For this review, take the finished solid that the model builds, in its own axes (mm). Give positions to 0.01 mm unless a question says otherwise; leave off trailing zeros. Write each loop counter-clockwise with the first axis right and the second up, starting at its lowest first coordinate (ties: lowest second). Pieces come first, ordered by that corner, then holes. Notation, with made-up numbers: M -30.75,37.25 L -25.75,37.25 A25 ccw -25.75,49.25 Z; hole C 39.25,-35 d7. An arc over 180 degrees is marked long. Write item = value, one per line.
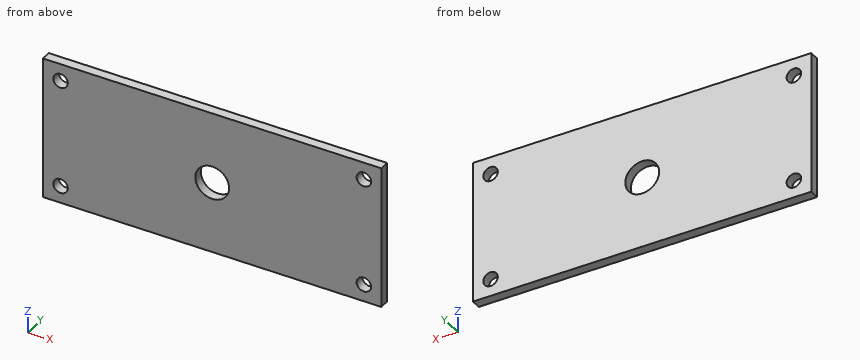
```python
from build123d import *

# Parameters (mm, degrees)
F0_W     = 70
F0_H     = 30
F1_DEPTH = 2
F2_R     = 1.5
F3_DEPTH = 25
F4_R     = 3.5
F5_DEPTH = 2.001


with BuildPart() as f1:
    # F0 (on Front) → F1 (new body)
    with BuildSketch(Plane.XZ):
        Rectangle(F0_W, F0_H)
    extrude(amount=F1_DEPTH)

    # F2 (on face) → F3 (cut)
    with BuildSketch(Plane.XZ.offset(2)):
        with Locations((-31.372793, 11.372793)):
            Circle(F2_R)
        with Locations((31.372793, 11.372793)):
            Circle(F2_R)
        with Locations((-31.372793, -11.372793)):
            Circle(F2_R)
        with Locations((31.372793, -11.372793)):
            Circle(F2_R)
    extrude(amount=-F3_DEPTH, mode=Mode.SUBTRACT)

    # F4 (on face) → F5 (cut, through all)
    with BuildSketch(Plane.XZ.offset(2)):
        Circle(F4_R)
    extrude(amount=-F5_DEPTH, mode=Mode.SUBTRACT)


solid = f1.part
```
1. Insertion check: P1, Ø5, axis at x = -31.37, z = -11.37, coming from the +Y side. The pin has a flat end and moves straight along its axis. Give the tip position at first contact, or say it passes through.
Responses:
P1 = 0
2. We need section D-D, the plane z = 10.75. Write out the cut boundary in (x, y).
Responses:
outline = M -35,-2 L -32.74,-2 L -32.74,0 L -35,0 Z; M -30.01,-2 L 30.01,-2 L 30.01,0 L -30.01,0 Z; M 32.74,-2 L 35,-2 L 35,0 L 32.74,0 Z
3. We need section B-B, the plane z = 0. Write out the cut boundary in (x, y).
Responses:
outline = M -35,-2 L -3.5,-2 L -3.5,0 L -35,0 Z; M 3.5,-2 L 35,-2 L 35,0 L 3.5,0 Z
4. We need section A-A, the plane x = 0. Write out the cut boundary in (y, z), then the cut area to 3 significant figures.
Responses:
outline = M -2,-15 L 0,-15 L 0,-3.5 L -2,-3.5 Z; M -2,3.5 L 0,3.5 L 0,15 L -2,15 Z
area = 46.0 mm2
5. For line 1 along X through (y, z) = (-0.5, 11.25); line 2 along X through (y, z) = (-1.45, 0.25); line 3 along X through (y, z) = (-1.75, -10.25), list the stretches that pass through material, from the lowest coordinate up. Write a range as from..to.
Responses:
line_1 = -35..-32.87, -29.88..29.88, 32.87..35
line_2 = -35..-3.49, 3.49..35
line_3 = -35..-32.37, -30.38..30.38, 32.37..35
6. We need section C-C, the plane y = -0.35. Write out the cut boundary in (x, z).
Responses:
outline = M -35,-15 L 35,-15 L 35,15 L -35,15 Z; hole C -31.37,-11.37 d3; hole C -31.37,11.37 d3; hole C 0,0 d7; hole C 31.37,-11.37 d3; hole C 31.37,11.37 d3
